```python
from build123d import *

# Parameters (mm, degrees)
SKETCH1_W                        = 24
SKETCH1_H                        = 39
BOSS_EXTRUDE1_DEPTH              = 10
F_10_0MM_DOWEL_HOLE1_D           = 10
F_10_0MM_DOWEL_HOLE1_DEPTH       = 24.5
F_10_0MM_DOWEL_HOLE1_CSINK_D     = 10.05
F_10_0MM_DOWEL_HOLE1_CSINK_ANGLE = 90
F_10_0MM_DOWEL_HOLE1_TIP         = 3.004303095
F_10_0MM_DOWEL_HOLE2_D           = 10
F_10_0MM_DOWEL_HOLE2_DEPTH       = 24.5
F_10_0MM_DOWEL_HOLE2_CSINK_D     = 10.05
F_10_0MM_DOWEL_HOLE2_CSINK_ANGLE = 90
F_10_0MM_DOWEL_HOLE2_TIP         = 3.004303095
FILLET1_R                        = 3


with BuildPart() as part:
    # Sketch1 → Boss-Extrude1 (new, symmetric)
    with BuildSketch(Plane.XY):
        Polygon((-18, -18.349478444), (-18, 18.349478444), (-12, 25.5), (12, 25.5), (18, 18.349478444), (18, -18.349478444), (12, -25.5), (-12, -25.5), align=None)
        Rectangle(SKETCH1_W, SKETCH1_H, mode=Mode.SUBTRACT)
    extrude(amount=BOSS_EXTRUDE1_DEPTH, both=True)

    # Ø10.0mm Dowel Hole1
    with Locations(Plane(origin=(0, 25.5, 0), x_dir=(1, 0, 0), z_dir=(0, 1, 0))):
        with Locations((0, 0)):
            CounterSinkHole(F_10_0MM_DOWEL_HOLE1_D / 2, F_10_0MM_DOWEL_HOLE1_CSINK_D / 2, depth=F_10_0MM_DOWEL_HOLE1_DEPTH, counter_sink_angle=F_10_0MM_DOWEL_HOLE1_CSINK_ANGLE)
            with Locations((0, 0, -(F_10_0MM_DOWEL_HOLE1_DEPTH + F_10_0MM_DOWEL_HOLE1_TIP / 2))):  # 118° drill point
                Cone(0, F_10_0MM_DOWEL_HOLE1_D / 2, F_10_0MM_DOWEL_HOLE1_TIP, mode=Mode.SUBTRACT)

    # Ø10.0mm Dowel Hole2
    with Locations(Plane(origin=(0, -25.5, 0), x_dir=(-1, 0, 0), z_dir=(0, -1, 0))):
        with Locations((0, 0)):
            CounterSinkHole(F_10_0MM_DOWEL_HOLE2_D / 2, F_10_0MM_DOWEL_HOLE2_CSINK_D / 2, depth=F_10_0MM_DOWEL_HOLE2_DEPTH, counter_sink_angle=F_10_0MM_DOWEL_HOLE2_CSINK_ANGLE)
            with Locations((0, 0, -(F_10_0MM_DOWEL_HOLE2_DEPTH + F_10_0MM_DOWEL_HOLE2_TIP / 2))):  # 118° drill point
                Cone(0, F_10_0MM_DOWEL_HOLE2_D / 2, F_10_0MM_DOWEL_HOLE2_TIP, mode=Mode.SUBTRACT)

    # Fillet1
    fillet1_edges = [part.edges().sort_by_distance(p)[0] for p in [
        (12, -19.5, 0),
        (12, 19.5, 0),
        (-12, 19.5, 0),
        (-12, -19.5, 0),
    ]]
    fillet(fillet1_edges, radius=FILLET1_R)


solid = part.part
```
Geometry check sheet. Reference: the model listing, model coordinates, mm. A direction names the side the tool comes from. Coordinates: 2 decimals unless noted, no trailing zeros. Write each loop counter-clockwise with the first axis right and the second up, starting at its lowest first coordinate (ties: lowest second). Pieces come first, ordered by that corner, then holes. Notation, with made-up numbers: M 39,55.5 L 53,55.5 A21 cw 53,94.5 Z; hole C 19.5,-30 d4. An arc over 180 degrees is marked long. Use one line per item in the form item = value. Start each with the question number.
1) Thickness scan on probe 1 along X at (y, z) = (12.5, 6.25); probe 2 along Y at (x, z) = (9, -0.25); probe 3 along Z at (x, y) = (0, 22.15). Record the ranges inside material, lowest first. Write a range as from..to.
2) Section check B-B on y = 9. Enter the section's corners in (x, z), and give its area (3 significant figures).
3) Section check C-C on z = -8. Enter the section's corners in (x, y).
4) Section check A-A on x = 0. Enter the section's corners in (y, z) (3 decimals), and give its area (3 significant figures).
5) Release check for a two-part mould opening along Z. For faces 3 (the flat face through (12.3, 0.4, -10)), 4 (the flat face through (-2, -19.5, 5)), 5 (the cylindrical face through (1.08, 22.45, 4.88)) record: pulls with the +Z half, pulls with the -Z half, needs draft (parallel to the pull), parting line crosses it, or undercut.
6) Set-up check for faces 1 (the flat face through (-2, 19.5, 5)), 2 (the flat face through (15.042, -21.875, 0.14)): record each of +Z, -Z, +X, -X, +Y, -Y from which the full face is reachable in a straight line by a thin tool's end or side.
7) Section check D-D on x = -7.5. Enter the section's corners in (y, z), and give its area (3 significant figures).
Responses:
q1.probe_1 = -18..-12, 12..18
q1.probe_2 = -25.5..-19.5, 19.5..25.5
q1.probe_3 = -10..-5, 5..10
q2.outline = M -18,-10 L -12,-10 L -12,10 L -18,10 Z; M 12,-10 L 18,-10 L 18,10 L 12,10 Z
q2.area = 240 mm2
q3.outline = M -18,-18.35 L -12,-25.5 L 12,-25.5 L 18,-18.35 L 18,18.35 L 12,25.5 L -12,25.5 L -18,18.35 Z; hole M -12,-16.5 A3 ccw -9,-19.5 L 9,-19.5 A3 ccw 12,-16.5 L 12,16.5 A3 ccw 9,19.5 L -9,19.5 A3 ccw -12,16.5 Z
q4.outline = M -25.5,-10 L -19.5,-10 L -19.5,-5 L -25.475,-5 L -25.5,-5.025 Z; M -25.5,5.025 L -25.475,5 L -19.5,5 L -19.5,10 L -25.5,10 Z; M 19.5,-10 L 25.5,-10 L 25.5,-5.025 L 25.475,-5 L 19.5,-5 Z; M 19.5,5 L 25.475,5 L 25.5,5.025 L 25.5,10 L 19.5,10 Z
q4.area = 120 mm2
q5.face_3 = pulls with the -Z half
q5.face_4 = needs draft
q5.face_5 = undercut
q6.face_1 = +Z, -Z
q6.face_2 = +Z, -Z, +X, -Y
q7.outline = M -25.5,-10 L -19.5,-10 L -19.5,10 L -25.5,10 Z; M 19.5,-10 L 25.5,-10 L 25.5,10 L 19.5,10 Z
q7.area = 240 mm2
